Design review of the part built by this model. Coordinates are the model's own, in mm. Coordinates: 2 decimals unless noted, no trailing zeros. Order: outer loops, then holes, each group sorted by start corner. A loop starts at its lowest first (then second) coordinate and runs counter-clockwise, first axis right, second up. Notation, with made-up numbers: M 4,35.5 L 10,35.5 A17 ccw 10,59.5 Z; hole C 6,69 d9. An arc over 180 degrees is marked long. Answer as a JSON object with one key per item and string values.
from build123d import *

# Parameters (mm, degrees)
SKETCH1_W           = 88.9
SKETCH1_H           = 88.9
BOSS_EXTRUDE1_DEPTH = 8.255
SKETCH5_W           = 88.9
SKETCH5_H           = 88.9
SKETCH5_R           = 41.91
CUT_EXTRUDE5_DEPTH  = 8.255
SKETCH9_R           = 4.191
CUT_EXTRUDE7_DEPTH  = 8.255
CIRPATTERN1_COUNT   = 4
CUT_EXTRUDE9_DEPTH  = 8.255
CIRPATTERN3_COUNT   = 6
SKETCH8_R           = 19.05
CUT_EXTRUDE10_DEPTH = 8.255


with BuildPart() as part:
    # Sketch1 → Boss-Extrude1 (new body)
    with BuildSketch(Plane(origin=(0, 0, 0), x_dir=(1, 0, 0), z_dir=(0, 1, 0))):
        with Locations((44.45, -44.45)):
            Rectangle(SKETCH1_W, SKETCH1_H)
    extrude(amount=-BOSS_EXTRUDE1_DEPTH)

    # Sketch5 → Cut-Extrude5 (cut)
    with BuildSketch(Plane(origin=(0, 0, 0), x_dir=(1, 0, 0), z_dir=(0, 1, 0))):
        with Locations((44.45, -44.45)):
            Rectangle(SKETCH5_W, SKETCH5_H)
        with Locations((44.45, -44.45)):
            Circle(SKETCH5_R, mode=Mode.SUBTRACT)
    extrude(amount=-CUT_EXTRUDE5_DEPTH, mode=Mode.SUBTRACT)

    # Sketch9 → Cut-Extrude7 (cut)
    with BuildSketch(Plane(origin=(0, 0, 0), x_dir=(1, 0, 0), z_dir=(0, 1, 0))):
        with Locations((44.45, -79.5528)):
            Circle(SKETCH9_R)
    cut_extrude7 = extrude(amount=-CUT_EXTRUDE7_DEPTH, mode=Mode.SUBTRACT)

    # CirPattern1: Cut-Extrude7 ×4 about axis
    cirpattern1_axis = Axis((44.45, 0, 44.45), (0, 1, 0))
    for i in range(1, CIRPATTERN1_COUNT):
        add(cut_extrude7.rotate(cirpattern1_axis, i * 360 / CIRPATTERN1_COUNT), mode=Mode.SUBTRACT)

    # Sketch11 → Cut-Extrude9 (cut)
    with BuildSketch(Plane(origin=(0, 0, 0), x_dir=(1, 0, 0), z_dir=(0, 1, 0))):
        with BuildLine():
            ThreePointArc((38.743889634, -67.945), (38.237051273, -66.340217261), (36.900419598, -65.317657467))
            Line((36.900419598, -65.317657467), (34.99935967, -70.572342533))
            ThreePointArc((34.99935967, -70.572342533), (37.554672374, -70.232161638), (38.743889634, -67.945))
        make_face()
        with BuildLine():
            Line((34.99935967, -70.572342533), (36.900419598, -65.317657467))
            ThreePointArc((36.900419598, -65.317657467), (33.322547101, -66.994470036), (34.99935967, -70.572342533))
        make_face()
    cut_extrude9 = extrude(amount=-CUT_EXTRUDE9_DEPTH, mode=Mode.SUBTRACT)

    # CirPattern3: Cut-Extrude9 ×6 about axis
    cirpattern3_axis = Axis((44.45, 0, 44.45), (0, 1, 0))
    for i in range(1, CIRPATTERN3_COUNT):
        add(cut_extrude9.rotate(cirpattern3_axis, i * 360 / CIRPATTERN3_COUNT), mode=Mode.SUBTRACT)

    # Sketch8 → Cut-Extrude10 (cut)
    with BuildSketch(Plane(origin=(0, 0, 0), x_dir=(1, 0, 0), z_dir=(0, 1, 0))):
        with Locations((44.45, -44.45)):
            Circle(SKETCH8_R)
    extrude(amount=-CUT_EXTRUDE10_DEPTH, mode=Mode.SUBTRACT)


solid = part.part
1) To check wall thickness, follow L1, parallel to X at y = -3.25, z = 48; L2, parallel to Z at x = 46, y = -5.5; L3, parallel to X at y = -2.5, z = 44.45. State the ranges of each line that lie inside material, in increasing order.
Taken from the geometry:
{"L1": "x = 2.69 to 7.12, 11.57 to 17.19, 22.52 to 25.73, 63.17 to 77.33, 81.78 to 86.21", "L2": "z = 2.57 to 5.45, 13.24 to 25.46, 63.44 to 75.66, 83.45 to 86.33", "L3": "x = 2.54 to 5.16, 13.54 to 25.4, 63.5 to 75.36, 83.74 to 86.36"}
2) Add section D-D (x = 69.5). State the section outline as (y, z) points (3 decimals).
Taken from the geometry:
{"outline": "M -8.255,10.85 L 0,10.85 L 0,37.307 L -8.255,37.307 Z; M -8.255,42.821 L 0,42.821 L 0,78.05 L -8.255,78.05 Z"}
3) Add section A-A (z = 44.45). State the section outline as (x, y) points (3 decimals).
Taken from the geometry:
{"outline": "M 2.54,-8.255 L 5.156,-8.255 L 5.156,0 L 2.54,0 Z; M 13.538,-8.255 L 25.4,-8.255 L 25.4,0 L 13.538,0 Z; M 63.5,-8.255 L 75.362,-8.255 L 75.362,0 L 63.5,0 Z; M 83.744,-8.255 L 86.36,-8.255 L 86.36,0 L 83.744,0 Z"}
4) Add section B-B (x = 44.45). State the section outline as (y, z) points (3 decimals).
Taken from the geometry:
{"outline": "M -8.255,2.54 L 0,2.54 L 0,5.156 L -8.255,5.156 Z; M -8.255,13.538 L 0,13.538 L 0,25.4 L -8.255,25.4 Z; M -8.255,63.5 L 0,63.5 L 0,75.362 L -8.255,75.362 Z; M -8.255,83.744 L 0,83.744 L 0,86.36 L -8.255,86.36 Z"}
5) Add section C-C (y = -4.5). Count the separate pieces of the cut face and the enclosed holes in it, and give its area (3 significant figures).
Taken from the geometry:
{"separate pieces": "1", "enclosed holes": "11", "area": "4,010 mm2"}
6) Insertion check: pin 1 Ø13.5 at (x, z) = (9.35, 44.45) entering from +Y; pin 2 Ø23 at (x, z) = (44.45, 44.45) entering from +Y; pin 3 Ø1.5 at (y, z) = (-3.5, 47) entering from +X; pin 4 Ø4 at (y, z) = (-1, 13.5) entering from -X. Each pin has a flat end and moves straight along its axis. Give the tip position at first contact, or say it passes through.
Taken from the geometry:
{"pin 1": "stops at y = 0", "pin 2": "passes through", "pin 3": "stops at x = 86.32", "pin 4": "stops at x = 14.15"}
7) Mouldability with a two-part tool opening along X and no side actions: class faces 1 (the flat face through (25, -8.255, 44)), 2 (the cylindrical face through (41.97, -4.07, 25.562)), 3 (the cylindrical face through (43.541, -4.07, 83.644)), 4 (the cylindrical face through (11.19, -4.07, 69.95)) as released by +X, released by -X, zero draft, split by the parting line, or undercut.
Taken from the geometry:
{"face 1": "zero draft", "face 2": "undercut", "face 3": "undercut", "face 4": "split by the parting line"}
